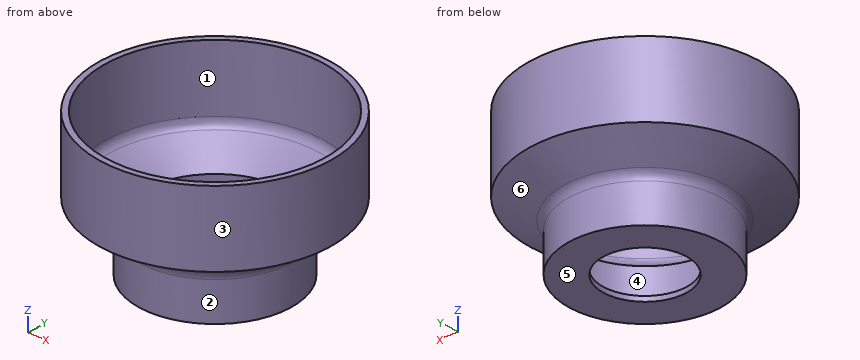
```python
from build123d import *


with BuildPart() as part:
    # Sketch1 → Revolve1 (revolve)
    with BuildSketch(Plane(origin=(0, 0, 0), x_dir=(1, 0, 0), z_dir=(0, 1, 0))):
        with BuildLine():
            Line((6.35, -0.762), (10.795, -0.762))
            Line((10.795, -0.762), (10.795, -7.112))
            Line((10.795, -7.112), (15.875, -10.044939367))
            ThreePointArc((15.875, -10.044939367), (16.432822715, -10.602762083), (16.637, -11.364762083))
            Line((16.637, -11.364762083), (16.637, -21.336))
            Line((16.637, -21.336), (17.526, -21.336))
            Line((17.526, -21.336), (17.526, -10.118262852))
            Line((17.526, -10.118262852), (12.319, -7.112))
            ThreePointArc((12.319, -7.112), (11.761177285, -6.554177285), (11.557, -5.792177285))
            Line((11.557, -5.792177285), (11.557, 0))
            Line((11.557, 0), (6.35, 0))
            Line((6.35, 0), (6.35, -0.762))
        make_face()
    revolve(axis=Axis((0, 0, 0), (0, 0, 1)))


solid = part.part
```
Geometry check sheet. Reference: the model listing, model coordinates, mm. Face numbers are marked on the shaded views. A direction names the side the tool comes from. Coordinates: 2 decimals unless noted, no trailing zeros. Order: outer loops, then holes, each group sorted by start corner. A loop starts at its lowest first (then second) coordinate and runs counter-clockwise, first axis right, second up. Notation, with made-up numbers: M 16,8.5 L 69,8.5 A23 cw 69,36.5 Z; hole C 72.25,0.25 d2. An arc over 180 degrees is marked long. Answer as a JSON object with one key per item and string values.
Q1. Release check for a two-part mould opening along Y. For the marked faces 4, 5 and 6 record: released by +Y, released by -Y, zero draft, split by the parting line, or undercut.
Results are:
{"face 4": "undercut", "face 5": "zero draft", "face 6": "split by the parting line"}
Q2. Scan lines: line 1 (Y direction, x = 0, z = 2.5) (3 decimals); line 2 (Y direction, x = 0, z = 0.2); line 3 (Z direction, x = -0.5, y = 10). Record each from-to range of solid material in increasing order.
Results are:
{"line 1": "y = -11.557 to -10.795, 10.795 to 11.557", "line 2": "y = -11.56 to -6.35, 6.35 to 11.56", "line 3": "z = 0 to 0.76"}
Q3. Tool access check on the marked faces 1, 2 and 3. Record the directions out of +Z, -Z, +X, -X, +Y, -Y that give a thin tool (end or side, any length) a straight path to the whole face; none if there is none.
Results are:
{"face 1": "+Z", "face 2": "-Z", "face 3": "+Z, -Z"}
Q4. Cross-section at D-D on z = 7.75. Record the cut outline in (x, y), and give its area (3 significant figures).
Results are:
{"outline": "C 0,0 d26.85; hole C 0,0 d23.8", "area": "121 mm²"}
Q5. Cross-section at C-C on z = 13.25. Record the cut outline in (x, y), and give its area (3 significant figures).
Results are:
{"outline": "C 0,0 d35.05; hole C 0,0 d33.27", "area": "95.4 mm²"}
Q6. Depth check by flat-ended pin: pin 1 Ø1.5 at (x, y) = (-9, -8) entering from +Z; pin 2 Ø14.5 at (x, y) = (0, 0) entering from +Z; pin 3 Ø2 at (x, y) = (13.5, 9) entering from -Z. Enter the tip coordinate at first touch or a pass-through.
Results are:
{"pin 1": "stops at z = 8.26", "pin 2": "stops at z = 0.76", "pin 3": "stops at z = 8.79"}
Q7. Cross-section at A-A on y = 0. Record the cut outline in (x, z) (3 decimals).
Results are:
{"outline": "M -17.526,10.118 L -12.319,7.112 A1.524 cw -11.557,5.792 L -11.557,0 L -6.35,0 L -6.35,0.762 L -10.795,0.762 L -10.795,7.112 L -15.875,10.045 A1.524 cw -16.637,11.365 L -16.637,21.336 L -17.526,21.336 Z; M 6.35,0 L 11.557,0 L 11.557,5.792 A1.524 cw 12.319,7.112 L 17.526,10.118 L 17.526,21.336 L 16.637,21.336 L 16.637,11.365 A1.524 cw 15.875,10.045 L 10.795,7.112 L 10.795,0.762 L 6.35,0.762 Z"}
